```python
from build123d import *

# Parameters (mm, degrees)
SKETCH1_W           = 25
SKETCH1_H           = 40
BOSS_EXTRUDE1_DEPTH = 1.5
SKETCH5_W           = 40
SKETCH5_H           = 25
BOSS_EXTRUDE3_DEPTH = 1.5
SKETCH6_W           = 50
SKETCH6_H           = 40
BOSS_EXTRUDE4_DEPTH = 1.5
SKETCH7_W           = 40
SKETCH7_H           = 26.5
BOSS_EXTRUDE5_DEPTH = 1.5
SKETCH9_W           = 25
SKETCH9_H           = 40
BOSS_EXTRUDE6_DEPTH = 1.5
FILLET2_R           = 3
SKETCH10_R          = 10
CUT_EXTRUDE1_DEPTH  = 1.5
FILLET3_R           = 3


with BuildPart() as part:
    # Sketch1 → Boss-Extrude1 (new body)
    with BuildSketch(Plane(origin=(0, 0, 0), x_dir=(1, 0, 0), z_dir=(0, 1, 0))):
        Rectangle(SKETCH1_W, SKETCH1_H)
    extrude(amount=BOSS_EXTRUDE1_DEPTH)

    # Sketch5 → Boss-Extrude3 (add)
    with BuildSketch(Plane(origin=(12.5, 0, 0), x_dir=(0, 0, -1), z_dir=(1, 0, 0))):
        with Locations((0, 12.5)):
            Rectangle(SKETCH5_W, SKETCH5_H)
    extrude(amount=BOSS_EXTRUDE3_DEPTH)

    # Sketch6 → Boss-Extrude4 (add)
    with BuildSketch(Plane(origin=(0, 25, 0), x_dir=(1, 0, 0), z_dir=(0, 1, 0))):
        with Locations((37.5, 0)):
            Rectangle(SKETCH6_W, SKETCH6_H)
    extrude(amount=BOSS_EXTRUDE4_DEPTH)

    # Sketch7 → Boss-Extrude5 (add)
    with BuildSketch(Plane(origin=(62.5, 0, 0), x_dir=(0, 0, -1), z_dir=(1, 0, 0))):
        with Locations((0, 13.25)):
            Rectangle(SKETCH7_W, SKETCH7_H)
    extrude(amount=BOSS_EXTRUDE5_DEPTH)

    # Sketch9 → Boss-Extrude6 (add)
    with BuildSketch(Plane(origin=(0, 0, 0), x_dir=(1, 0, 0), z_dir=(0, 1, 0))):
        with Locations((76.5, 0)):
            Rectangle(SKETCH9_W, SKETCH9_H)
    extrude(amount=BOSS_EXTRUDE6_DEPTH)

    # Fillet2
    fillet2_edges = [part.edges().sort_by_distance(p)[0] for p in [
        (14, 0, 0),
        (12.5, 26.5, 0),
        (62.5, 0, 0),
        (64, 26.5, 0),
    ]]
    fillet(fillet2_edges, radius=FILLET2_R)

    # Sketch10 → Cut-Extrude1 (cut)
    with BuildSketch(Plane(origin=(0, 26.5, 0), x_dir=(1, 0, 0), z_dir=(0, 1, 0))):
        with Locations(Location((38.25, 0, 0), (0, 0, 270))):
            Circle(SKETCH10_R)
    extrude(amount=-CUT_EXTRUDE1_DEPTH, mode=Mode.SUBTRACT)

    # Fillet3
    fillet3_edges = [part.edges().sort_by_distance(p)[0] for p in [
        (12.5, 1.5, 0),
        (64, 1.5, 0),
    ]]
    fillet(fillet3_edges, radius=FILLET3_R)


solid = part.part
```
Check sheet for the modelled part. Datum: model origin and axes. Units: mm. A direction names the side the tool comes from. Coordinates: 2 decimals unless noted, no trailing zeros. Loops run counter-clockwise (first coordinate to the right, second up) from the corner with the lowest first, then second, coordinate; pieces in that order, holes last. Notation, with made-up numbers: M 51,7.5 L 87,7.5 A19 cw 87,34.5 Z; hole C -2.75,-15.75 d11. An arc over 180 degrees is marked long. Answer as a JSON object with one key per item and string values.
1. Sectioned sample at A-A on z = 0. Record the cut outline in (x, y), and give its area (3 significant figures).
Outcome:
{"outline": "M -12.5,0 L 11,0 A3 ccw 14,3 L 14,25 L 28.25,25 L 28.25,26.5 L 15.5,26.5 A3 ccw 12.5,23.5 L 12.5,4.5 A3 cw 9.5,1.5 L -12.5,1.5 Z; M 48.25,25 L 62.5,25 L 62.5,3 A3 ccw 65.5,0 L 89,0 L 89,1.5 L 67,1.5 A3 cw 64,4.5 L 64,23.5 A3 ccw 61,26.5 L 48.25,26.5 Z", "area": "193 mm²"}
2. Sectioned sample at B-B on x = 38.25. Record the cut outline in (y, z), and give its area (3 significant figures).
Outcome:
{"outline": "M 25,-20 L 26.5,-20 L 26.5,-10 L 25,-10 Z; M 25,10 L 26.5,10 L 26.5,20 L 25,20 Z", "area": "30.0 mm²"}
3. Release check for a two-part mould opening along X. For faces 1 (the cylindrical face through (11.64, 2.4, -0.28)), 2 (the flat face through (-2, 1.5, 0)), 3 (the flat face through (14, 14, 0)), 4 (the cylindrical face through (13.1, 0.86, -0.28)) record: pulls with the +X half, pulls with the -X half, needs draft (parallel to the pull), parting line crosses it, or undercut.
Outcome:
{"face 1": "pulls with the -X half", "face 2": "needs draft", "face 3": "undercut", "face 4": "undercut"}
4. Depth check by flat-ended pin: P1, Ø6, axis at y = 22.5, z = 4.5, coming from the +X side; P2, Ø17.5, axis at x = 73.5, z = -5, coming from the +Y side; P3, Ø1, axis at x = 60.5, y = 20, coming from the +Z side; P4, Ø9.5, axis at y = 17, z = -0.5, coming from the -X side. Enter the tip coordinate at first touch or a pass-through.
Outcome:
{"P1": "x = 64", "P2": "y = 2.52", "P3": "through", "P4": "x = 12.5"}
5. Sectioned sample at C-C on y = 21. Record the cut outline in (x, z).
Outcome:
{"outline": "M 12.5,-20 L 14,-20 L 14,20 L 12.5,20 Z; M 62.5,-20 L 64,-20 L 64,20 L 62.5,20 Z"}
6. Scan lines: L1, parallel to X at y = 5.25, z = 4.5; L2, parallel to Y at x = 54, z = 6.5; L3, parallel to Y at x = 1.5, z = -8. Record each from-to range of solid material in increasing order. Write a range as from..to.
Outcome:
{"L1": "12.5..14, 62.5..64", "L2": "25..26.5", "L3": "0..1.5"}
7. Access from +Z, -Z, +X, -X, +Y, -Y to the whole of each face (thin tool, end or side, straight path). Record for faces 5 (the cylindrical face through (63.36, 0.9, -0.28)), 6 (the flat face through (12.5, 14, 0)), 7 (the flat face through (78, 1.5, 0)).
Outcome:
{"face 5": "+Z, -Z, -Y", "face 6": "+Z, -Z, -X, +Y", "face 7": "+Z, -Z, +X, +Y"}
8. Sectioned sample at D-D on z = -15. Record the cut outline in (x, y), and give its area (3 significant figures).
Outcome:
{"outline": "M -12.5,0 L 11,0 A3 ccw 14,3 L 14,25 L 62.5,25 L 62.5,3 A3 ccw 65.5,0 L 89,0 L 89,1.5 L 67,1.5 A3 cw 64,4.5 L 64,23.5 A3 ccw 61,26.5 L 15.5,26.5 A3 ccw 12.5,23.5 L 12.5,4.5 A3 cw 9.5,1.5 L -12.5,1.5 Z", "area": "223 mm²"}
